from build123d import *

# Parameters (mm, degrees)
SKETCH2_R                = 3
SKETCH2_R_2              = 1.7
BOSS_EXTRUDE1_DEPTH      = 1
SKETCH3_W                = 3
SKETCH3_H                = 1
BOSS_EXTRUDE2_DEPTH      = 5
BOSS_EXTRUDE3_DEPTH      = 1
BOSS_EXTRUDE3_DEPTH_BACK = 1
FILLET1_R                = 1


with BuildPart() as part:
    # Sketch2 → Boss-Extrude1 (new body)
    with BuildSketch(Plane(origin=(0, 0, 0), x_dir=(1, 0, 0), z_dir=(0, 1, 0))):
        with BuildLine():
            ThreePointArc((-12.345669291, -2.979001468), (12.7, 0), (-12.345669291, 2.979001468))
            ThreePointArc((-12.345669291, 2.979001468), (-15.7, 0), (-12.345669291, -2.979001468))
        make_face()
        with Locations(Location((0, 0, 0), (0, 0, 270))):
            Circle(SKETCH2_R, mode=Mode.SUBTRACT)
        with Locations(Location((-12.7, 0, 0), (0, 0, 270))):
            Circle(SKETCH2_R_2, mode=Mode.SUBTRACT)
    extrude(amount=BOSS_EXTRUDE1_DEPTH)

    # Sketch3 → Boss-Extrude2 (add)
    with BuildSketch(Plane(origin=(0, 1, 0), x_dir=(1, 0, 0), z_dir=(0, 1, 0))):
        with Locations((0, 6.75)):
            Rectangle(SKETCH3_W, SKETCH3_H)
        with Locations((0, -6.75)):
            Rectangle(SKETCH3_W, SKETCH3_H)
    extrude(amount=BOSS_EXTRUDE2_DEPTH)

    # Sketch4 → Boss-Extrude3 (add, two sides: drawn at the far end of the back side and taken through both)
    with BuildSketch(Plane(origin=(0, 0, 0), x_dir=(0, 0, -1), z_dir=(1, 0, 0)).offset(-BOSS_EXTRUDE3_DEPTH_BACK)):
        Polygon((-6.25, 4.75), (-5.25, 3.75), (-5.25, 3.25), (-6.25, 3.25), align=None)
        Polygon((5.25, 3.75), (6.25, 4.75), (6.25, 3.25), (5.25, 3.25), align=None)
    extrude(amount=BOSS_EXTRUDE3_DEPTH + BOSS_EXTRUDE3_DEPTH_BACK)

    # Fillet1
    fillet1_edges = [part.edges().sort_by_distance(p)[0] for p in [
        (-1.5, 1, -6.75),
        (1.5, 1, -6.75),
        (0, 1, -7.25),
        (-1.5, 1, 6.75),
        (0, 1, 7.25),
        (1.5, 1, 6.75),
    ]]
    fillet(fillet1_edges, radius=FILLET1_R)


solid = part.part
The listing builds one solid part. Answer for the finished solid, in the listing's coordinates (mm). A direction names the side the tool comes from. Round coordinates to 2 decimals unless told otherwise and drop trailing zeros. Order: outer loops, then holes, each group sorted by start corner. A loop starts at its lowest first (then second) coordinate and runs counter-clockwise, first axis right, second up. Notation, with made-up numbers: (21.25, -24.5) -> (59.25, -24.5) arc R27 ccw to (59.25, 3.5) -> close; hole circle Ø8 at (79.25, -13.5). An arc over 180 degrees is marked (long way). Put each result on its own line as item: value.
Q1. Section B-B, the plane y = 2.85 is taken. Write down the section's boundary in (x, z).
Results list:
outline: (-1.5, -7.25) -> (1.5, -7.25) -> (1.5, -6.25) -> (-1.5, -6.25) -> close; (-1.5, 6.25) -> (1.5, 6.25) -> (1.5, 7.25) -> (-1.5, 7.25) -> close
Q2. Section A-A, the plane x = 0 is taken. Write down the section's boundary in (y, z), and give its area (3 significant figures).
Results list:
outline: (0, -12.7) -> (1, -12.7) -> (1, -8.25) arc R1 cw to (2, -7.25) -> (6, -7.25) -> (6, -6.25) -> (4.75, -6.25) -> (3.75, -5.25) -> (3.25, -5.25) -> (3.25, -6.25) -> (1, -6.25) -> (1, -3) -> (0, -3) -> close; (0, 3) -> (1, 3) -> (1, 6.25) -> (3.25, 6.25) -> (3.25, 5.25) -> (3.75, 5.25) -> (4.75, 6.25) -> (6, 6.25) -> (6, 7.25) -> (2, 7.25) arc R1 cw to (1, 8.25) -> (1, 12.7) -> (0, 12.7) -> close
area: 31.8 mm^2
Q3. Section D-D, the plane x = -12.7 is taken. Write down the section's boundary in (y, z), and give its area (3 significant figures).
Results list:
outline: (0, -3) -> (1, -3) -> (1, -1.7) -> (0, -1.7) -> close; (0, 1.7) -> (1, 1.7) -> (1, 3) -> (0, 3) -> close
area: 2.60 mm^2
Q4. Determine the mould class of faces 6 (the flat face through (-1.5, 4, 7)), 7 (the flat face through (0, 4.2, -5.7)), 8 (the cylindrical face through (-11.014, 0.493, -0.221)), 9 (the cylindrical face through (0.9, 0.49, 2.86)) for opening direction X: pulls with the +X half, pulls with the -X half, needs draft (parallel to the pull), parting line crosses it, or undercut.
Results list:
face 6: pulls with the -X half
face 7: needs draft
face 8: undercut
face 9: undercut
Q5. Consider line 1 along Y through (x, z) = (-11, -3.75); line 2 along X through (y, z) = (1.85, 7); line 3 along X through (y, z) = (0.45, -9). Determine where each line is inside the solid, lowest interval first.
Results list:
line 1: 0 to 1
line 2: -1.51 to 1.51
line 3: -8.96 to 8.96
Q6. Which of the six approach directions +Z, -Z, +X, -X, +Y, -Y give full straight-line access (tool end or side, diameter ignored) to faces 1 (the flat face through (1, 4, -6)), 2 (the flat face through (0, 3.25, 6)), 3 (the flat face through (1.5, 4, -7)), 4 (the flat face through (-1, 4, -6)), 5 (the flat face through (-1.5, 4, -7))?
Results list:
face 1: +X, +Y
face 2: +X, -X
face 3: +Z, -Z, +X, +Y
face 4: -X, +Y
face 5: +Z, -Z, -X, +Y
Q7. Section C-C, the plane z = 0 is taken. Write down the section's boundary in (x, y), and give its area (3 significant figures).
Results list:
outline: (-15.7, 0) -> (-14.4, 0) -> (-14.4, 1) -> (-15.7, 1) -> close; (-11, 0) -> (-3, 0) -> (-3, 1) -> (-11, 1) -> close; (3, 0) -> (12.7, 0) -> (12.7, 1) -> (3, 1) -> close
area: 19.0 mm^2
Q8. Each of these flat-tipped pins is pushed along its axis until it touches: P1, Ø0.6, axis at x = 0.5, y = 3.5, coming from the +Z side; P2, Ø1.1, axis at y = 3, z = 6.5, coming from the -X side; P3, Ø10, axis at x = 8.5, z = -5, coming from the +Y side. Where does it stop, or does it pass through?
Results list:
P1: z = 7.25
P2: x = -1.5
P3: y = 1
